Can you work these out from the drawing? Everything is in mm from the part's minimum corner. Give positions to 0.01 mm unless a question says otherwise; leave off trailing zeros. Order: outer loops, then holes, each group sorted by start corner. A loop starts at its lowest first (then second) coordinate and runs counter-clockwise, first axis right, second up. Notation, with made-up numbers: (36.25, 58.25) - (40.25, 58.25) arc R5 cw to (40.25, 66.25) - close; hole circle Ø5 at (86.25, -27.5). An arc over 180 degrees is marked (long way). One line per question, with ' | ' between items.
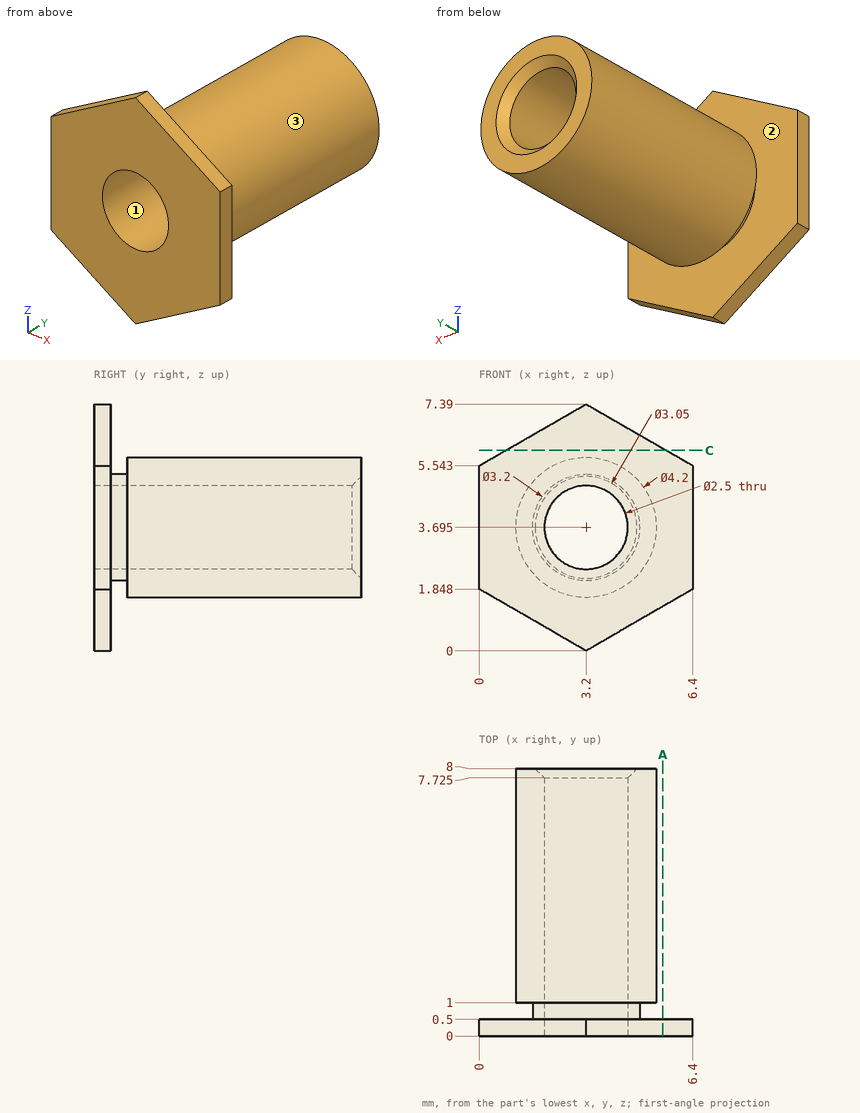
1) I want a section at C-C (z = 6). List the corners of the cut face in (x, y) for me.
Model answer:
outline: (0.79, 0) - (5.61, 0) - (5.61, 0.5) - (0.79, 0.5) - close
2) Please list where these lines run through material, in increasing order: L1, parallel to Z at x = 3.25, y = 3.25 (1 decimal); L2, parallel to X at y = 6.5, z = 2.25 (1 decimal); L3, parallel to X at y = 2.75, z = 4.25 (1 decimal).
Model answer:
L1: z = 1.6 to 2.4, 4.9 to 5.8 | L2: x = 1.7 to 4.7 | L3: x = 1.2 to 2.1, 4.3 to 5.2
3) I want a section at A-A (x = 5.5). List the corners of the cut face in (y, z) for me.
Model answer:
outline: (0, 1.33) - (0.5, 1.33) - (0.5, 6.06) - (0, 6.06) - close
4) I'm going to push flat-ended pins straight in: P1, Ø3, axis at x = 2, y = 4, coming from the -Z side (1 decimal); P2, Ø1.5, axis at x = 3.2, z = 3.7, coming from the -Y side. Where does each tip first touch, or does it pass through?
Model answer:
P1: stops at z = 1.6 | P2: passes through
5) Thinking about a two-plate mould opening in X: for the marked faces 1, 2 and 3, which applies, +X half, -X half, draft (parallel to the pull), parting line (faces both ways), or undercut?
Model answer:
face 1: undercut | face 2: draft | face 3: parting line
